Verification items for the finished model (mm, model axes). Face numbers are marked on the shaded views. A direction names the side the tool comes from. Round coordinates to 2 decimals unless told otherwise and drop trailing zeros. Write each loop counter-clockwise with the first axis right and the second up, starting at its lowest first coordinate (ties: lowest second). Pieces come first, ordered by that corner, then holes. Notation, with made-up numbers: M -14,-14.5 L 34,-14.5 A22 cw 34,-6.5 Z; hole C 73.25,1.5 d7. An arc over 180 degrees is marked long. Write each question's results on one line, items separated by ' | '.
from build123d import *

# Parameters (mm, degrees)
F0_W      = 28
F0_H      = 16
F1_DEPTH  = 8
F2_R      = 4
F3_DEPTH  = 4
F4_R      = 2.85
F5_DEPTH  = 1.5
F6_R      = 2.25
F7_DEPTH  = 25
F8_R      = 3
F10_DEPTH = 3
F9_R      = 3
F11_DEPTH = 3
F12_R     = 1.6
F14_DEPTH = 25
F13_R     = 1.6
F15_DEPTH = 25
F16_SIZE  = 0.5


with BuildPart() as f1:
    # F0 (on Front) → F1 (new body)
    with BuildSketch(Plane.XZ):
        with Locations((14, 8)):
            Rectangle(F0_W, F0_H)
    extrude(amount=F1_DEPTH)

    # F2 (on face) → F3 (cut)
    with BuildSketch(Plane.XZ.offset(8)):
        with Locations((14, 8)):
            Circle(F2_R)
    extrude(amount=-F3_DEPTH, mode=Mode.SUBTRACT)

    # F4 (on face) → F5 (cut)
    with BuildSketch(Plane.XZ.offset(4)):
        with Locations((14, 8)):
            Circle(F4_R)
    extrude(amount=-F5_DEPTH, mode=Mode.SUBTRACT)

    # F6 (on face) → F7 (cut)
    with BuildSketch(Plane.XZ.offset(2.5)):
        with Locations((14, 8)):
            Circle(F6_R)
    extrude(amount=-F7_DEPTH, mode=Mode.SUBTRACT)

    # F8 (on face) → F10 (cut)
    with BuildSketch(Plane.XY.offset(16)):
        with Locations((6, -4)):
            Circle(F8_R)
    extrude(amount=-F10_DEPTH, mode=Mode.SUBTRACT)

    # F9 (on face) → F11 (cut)
    with BuildSketch(Plane.XY.offset(16)):
        with Locations((22, -4)):
            Circle(F9_R)
    extrude(amount=-F11_DEPTH, mode=Mode.SUBTRACT)

    # F12 (on face) → F14 (cut)
    with BuildSketch(Plane.XY.offset(13)):
        with Locations((6, -4)):
            Circle(F12_R)
    extrude(amount=-F14_DEPTH, mode=Mode.SUBTRACT)

    # F13 (on face) → F15 (cut)
    with BuildSketch(Plane.XY.offset(13)):
        with Locations((22, -4)):
            Circle(F13_R)
    extrude(amount=-F15_DEPTH, mode=Mode.SUBTRACT)

    # F16
    f16_edges = [f1.edges().sort_by_distance(p)[0] for p in [
        (28, -8, 8),
        (28, -4, 16),
        (28, 0, 8),
        (14, -8, 16),
        (14, 0, 16),
        (0, -4, 16),
        (0, -8, 8),
        (0, 0, 8),
    ]]
    chamfer(f16_edges, length=F16_SIZE)


solid = f1.part
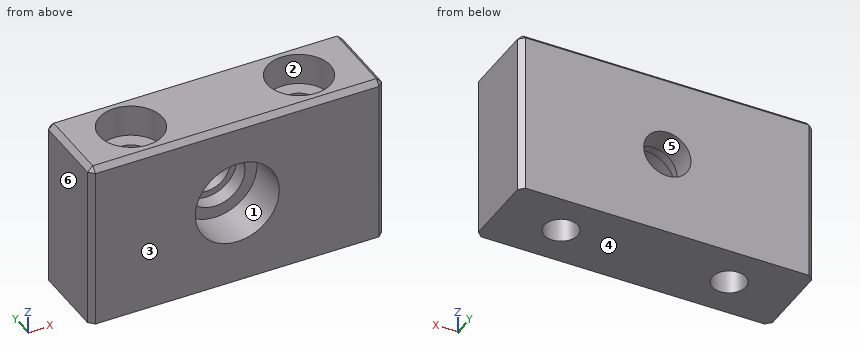
1) Depth check by flat-ended pin: P1, Ø1.9, axis at x = 22, y = -4, coming from the +Z side; P2, Ø2.5, axis at x = 15, z = 10, coming from the -Y side. Enter the tip coordinate at first touch or a pass-through.
Calculated:
P1: passes through | P2: stops at y = -4
2) Access from +Z, -Z, +X, -X, +Y, -Y to the whole of each face (thin tool, end or side, straight path). Record for the marked faces 1, 2 and 3.
Calculated:
face 1: -Y | face 2: +Z | face 3: +Z, -Z, +X, -X, -Y
3) Sectioned sample at A-A, the plane z = 8. Record the cut outline in (x, y).
Calculated:
outline: M 0,-7.5 L 0.5,-8 L 10,-8 L 10,-4 L 11.15,-4 L 11.15,-2.5 L 11.75,-2.5 L 11.75,0 L 0.5,0 L 0,-0.5 Z; M 16.25,-2.5 L 16.85,-2.5 L 16.85,-4 L 18,-4 L 18,-8 L 27.5,-8 L 28,-7.5 L 28,-0.5 L 27.5,0 L 16.25,0 Z; hole C 6,-4 d3.2; hole C 22,-4 d3.2
4) Sectioned sample at C-C, the plane z = 1. Record the cut outline in (x, y), and give its area (3 significant figures).
Calculated:
outline: M 0,-7.5 L 0.5,-8 L 27.5,-8 L 28,-7.5 L 28,-0.5 L 27.5,0 L 0.5,0 L 0,-0.5 Z; hole C 6,-4 d3.2; hole C 22,-4 d3.2 | area: 207 mm²
5) Sectioned sample at B-B, the plane x = 22. Record the cut outline in (y, z), and give its area (4 significant figures).
Calculated:
outline: M -8,0 L -5.6,0 L -5.6,13 L -7,13 L -7,16 L -7.5,16 L -8,15.5 Z; M -2.4,0 L 0,0 L 0,15.5 L -0.5,16 L -1,16 L -1,13 L -2.4,13 Z | area: 68.15 mm²
6) Material ranges on line 1 (Y direction, x = 22, z = 9.5); line 2 (Y direction, x = 6, z = 14.3); line 3 (Z direction, x = 14, y = -0.6), recorded low to high. Write a range as [from, to].
Calculated:
line 1: y = [-8, -5.6], [-2.4, 0] | line 2: y = [-8, -7], [-1, 0] | line 3: z = [0, 5.75], [10.25, 16]
7) Draft check along Z on the marked faces 4, 5 and 6. Enter one of: pulls with the +Z half, pulls with the -Z half, needs draft (parallel to the pull), parting line crosses it, or undercut.
Calculated:
face 4: pulls with the -Z half | face 5: undercut | face 6: needs draft
8) Sectioned sample at D-D, the plane y = -1.5. Record the cut outline in (x, z), and give its area (3 significant figures).
Calculated:
outline: M 0,0 L 28,0 L 28,15.5 L 27.5,16 L 23.66,16 L 23.66,13 L 20.34,13 L 20.34,16 L 7.66,16 L 7.66,13 L 4.34,13 L 4.34,16 L 0.5,16 L 0,15.5 Z; hole C 14,8 d4.5 | area: 412 mm²
